from build123d import *

# Parameters (mm, degrees)
SKETCH1_W                = 25.4
SKETCH1_H                = 25.4
SKETCH1_W_2              = 19.05
SKETCH1_H_2              = 19.05
BOSS_EXTRUDE1_DEPTH      = 254
F_0_257_DIAMETER_HOLE1_D = 6.5278


with BuildPart() as part:
    # Sketch1 → Boss-Extrude1 (new body)
    with BuildSketch(Plane.XY):
        Rectangle(SKETCH1_W, SKETCH1_H)
        Rectangle(SKETCH1_W_2, SKETCH1_H_2, mode=Mode.SUBTRACT)
    extrude(amount=BOSS_EXTRUDE1_DEPTH)

    # F (0.257) Diameter Hole1 (through all)
    with Locations(Plane(origin=(12.7, 0, 0), x_dir=(0, 0, -1), z_dir=(1, 0, 0))):
        with Locations((-215.9, 0), (-38.1, 0)):
            Hole(F_0_257_DIAMETER_HOLE1_D / 2)


solid = part.part
Could you check a few things on this model? Use its own coordinates, in mm. A direction names the side the tool comes from. Round coordinates to 2 decimals unless told otherwise and drop trailing zeros. Write each loop counter-clockwise with the first axis right and the second up, starting at its lowest first coordinate (ties: lowest second). Pieces come first, ordered by that corner, then holes. Notation, with made-up numbers: (38, -29) - (95, -29) arc R23 cw to (95, 0) - close; hole circle Ø2 at (-16.75, 38.5). An arc over 180 degrees is marked (long way). Use a Markdown table: item, result.
Q1. Thinking about a two-plate mould opening in Y: for faces 3 (the flat face through (11, 0, 254)), 4 (the flat face through (0, 12.7, 125)), 5 (the flat face through (9.525, 0, 125)), which applies, released by +Y, released by -Y, zero draft, split by the parting line, or undercut?
Output values:
| item | result |
|---|---|
| face 3 | zero draft |
| face 4 | released by +Y |
| face 5 | undercut |
Q2. For faces 1 (the flat face through (0, -9.525, 125)), 2 (the cylindrical face through (11.09, 0.14, 212.64)), which set-ups out of +Z, -Z, +X, -X, +Y, -Y let a thin tool reach every point of the face, with its end or its side?
Output values:
| item | result |
|---|---|
| face 1 | +Z, -Z |
| face 2 | +X, -X |
Q3. I want a section at D-D (z = 38.1). List the corners of the cut face in (x, y) for me (3 decimals).
Output values:
| item | result |
|---|---|
| outline | (-12.7, -12.7) - (12.7, -12.7) - (12.7, -3.264) - (9.525, -3.264) - (9.525, -9.525) - (-9.525, -9.525) - (-9.525, -3.264) - (-12.7, -3.264) - close; (-12.7, 3.264) - (-9.525, 3.264) - (-9.525, 9.525) - (9.525, 9.525) - (9.525, 3.264) - (12.7, 3.264) - (12.7, 12.7) - (-12.7, 12.7) - close |
Q4. Please list where these lines run through material, in increasing order: L1, parallel to Y at x = -11.5, z = 215.9; L2, parallel to X at y = 7.75, z = 170 (3 decimals).
Output values:
| item | result |
|---|---|
| L1 | -12.7 to -3.26, 3.26 to 12.7 |
| L2 | -12.7 to -9.525, 9.525 to 12.7 |
Q5. For pin 1 (6 mm diameter, centred on y = 0, z = 215.9, fed in from +X), with a flat end and sliding along its axis, tell me the tip position at first contact or that it passes through.
Output values:
| item | result |
|---|---|
| pin 1 | through |
Q6. I want a section at B-B (x = 3.5). List the corners of the cut face in (y, z) for me (3 decimals).
Output values:
| item | result |
|---|---|
| outline | (-12.7, 0) - (-9.525, 0) - (-9.525, 254) - (-12.7, 254) - close; (9.525, 0) - (12.7, 0) - (12.7, 254) - (9.525, 254) - close |
Q7. I want a section at A-A (z = 101). List the corners of the cut face in (x, y) for me (3 decimals), plus the area to 3 significant figures.
Output values:
| item | result |
|---|---|
| outline | (-12.7, -12.7) - (12.7, -12.7) - (12.7, 12.7) - (-12.7, 12.7) - close; hole (-9.525, -9.525) - (9.525, -9.525) - (9.525, 9.525) - (-9.525, 9.525) - close |
| area | 282 mm2 |
